Source: three-view drawing plus pictorial views. Frame: mm from the lowest corner of the part. A direction names the side the tool comes from. Round coordinates to 2 decimals unless told otherwise and drop trailing zeros. Order: outer loops, then holes, each group sorted by start corner. A loop starts at its lowest first (then second) coordinate and runs counter-clockwise, first axis right, second up. Notation, with made-up numbers: (-31.5, -40) - (0.5, -40) arc R19 ccw to (0.5, -8) - close; hole circle Ø3 at (16, 9.5). An arc over 180 degrees is marked (long way). Use one line per item in the form item = value. Start each with the question number.
Q1. Cut plane B-B, the plane x = 32. Return the cut outline in (y, z), and give its area (3 significant figures).
Q2. Cut plane D-D, the plane x = 59.5. Return the cut outline in (y, z).
Q3. Pin query (flat end, axial travel): pin 1 Ø7.5 at (y, z) = (118.5, 35) entering from -X; pin 2 Ø7.5 at (x, y) = (57.5, 59) entering from +Z; pin 3 Ø2 at (x, y) = (36.5, 101.5) entering from +Z. Return the tip coordinate at first contact, or that it passes through.
Q4. Cut plane A-A, the plane y = 137.5. Return the cut outline in (x, z), and give its area (3 significant figures).
Q5. Ray query, line 1 (Y direction, x = 52, z = 36.5); line 2 (X direction, y = 38.5, z = 43). Return the intervals inside material, ascending. Write a range as [from, to].
Q6. Set-up query: the marked faces 1, 2 and 3. Return all of +Z, -Z, +X, -X, +Y, -Y with unobstructed straight access to the full face (end or side cutting, diameter ignored); none if empty.
Q7. Cut plane C-C, the plane z = 39.5. Return the cut outline in (x, y).
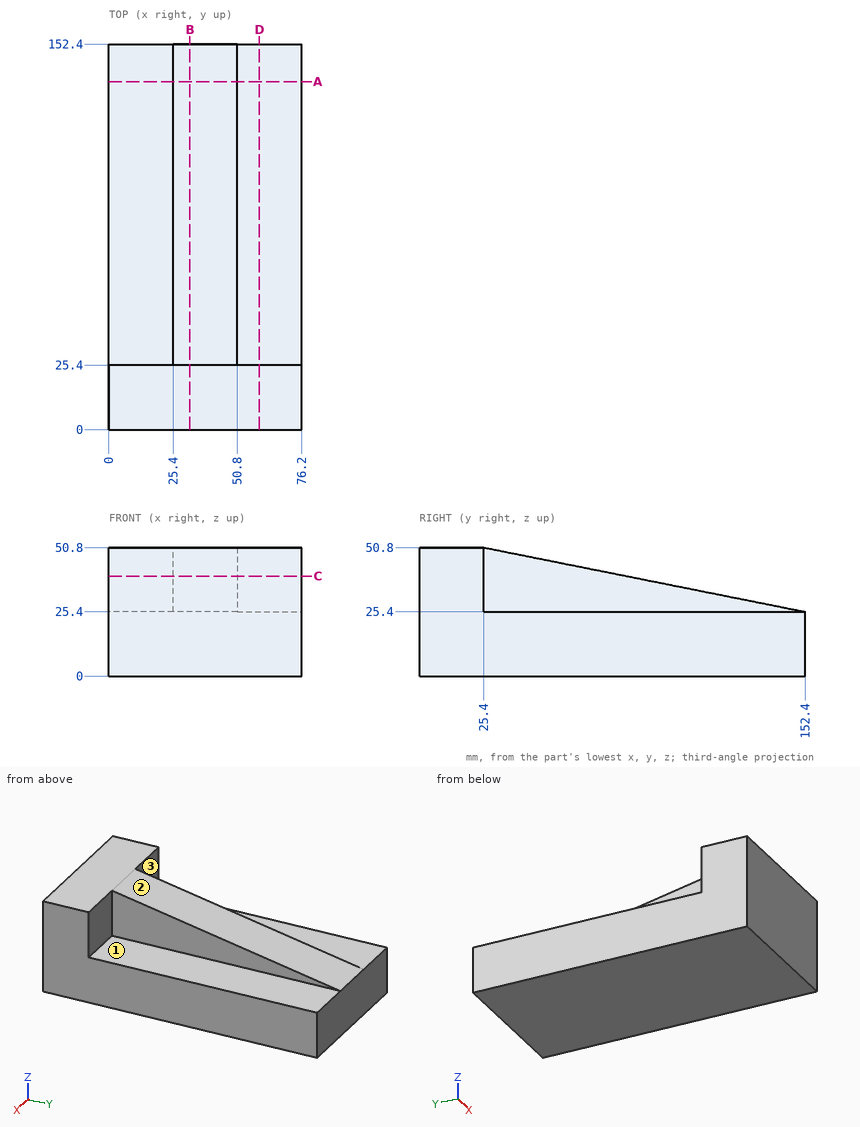
Completed:
q1.outline = (0, 0) - (152.4, 0) - (152.4, 25.4) - (25.4, 50.8) - (0, 50.8) - close
q1.area = 6,130 mm2
q2.outline = (0, 0) - (152.4, 0) - (152.4, 25.4) - (25.4, 25.4) - (25.4, 50.8) - (0, 50.8) - close
q3.pin_1 = 25.4
q3.pin_2 = 25.4
q3.pin_3 = 35.78
q4.outline = (0, 0) - (76.2, 0) - (76.2, 25.4) - (50.8, 25.4) - (50.8, 28.38) - (25.4, 28.38) - (25.4, 25.4) - (0, 25.4) - close
q4.area = 2,010 mm2
q5.line_1 = [0, 25.4]
q5.line_2 = [25.4, 50.8]
q6.face_1 = +Z, +X, +Y
q6.face_2 = +Z, +X, -X, +Y
q6.face_3 = +Z, -X, +Y
q7.outline = (0, 0) - (76.2, 0) - (76.2, 25.4) - (50.8, 25.4) - (50.8, 81.9) - (25.4, 81.9) - (25.4, 25.4) - (0, 25.4) - close
